from build123d import *

# Parameters (mm, degrees)
F0_R     = 11
F0_R_2   = 10
F0_R_3   = 8.75
F0_R_4   = 7.25
F0_R_5   = 3.5
F0_R_6   = 2.75
F1_DEPTH = 2
F2_DEPTH = 4.25
F3_DEPTH = 12


with BuildPart() as f1:
    # F0 (on Top) → F1 (new body)
    with BuildSketch(Plane.XY):
        Circle(F0_R)
        Circle(F0_R_2, mode=Mode.SUBTRACT)
        Circle(F0_R_2)
        Circle(F0_R_3, mode=Mode.SUBTRACT)
        Circle(F0_R_3)
        Circle(F0_R_4, mode=Mode.SUBTRACT)
        Circle(F0_R_4)
        Circle(F0_R_5, mode=Mode.SUBTRACT)
        Circle(F0_R_5)
        Circle(F0_R_6, mode=Mode.SUBTRACT)
    extrude(amount=F1_DEPTH)

    # F0 (on Top) → F2 (join)
    with BuildSketch(Plane.XY):
        Circle(F0_R_5)
        Circle(F0_R_6, mode=Mode.SUBTRACT)
    extrude(amount=-F2_DEPTH)

    # F0 (on Top) → F3 (join)
    with BuildSketch(Plane.XY):
        Circle(F0_R_2)
        Circle(F0_R_3, mode=Mode.SUBTRACT)
    extrude(amount=F3_DEPTH)


solid = f1.part
Part model, mm, in its own coordinate system. A direction names the side the tool comes from. Coordinates: 2 decimals unless noted, no trailing zeros. Order: outer loops, then holes, each group sorted by start corner. A loop starts at its lowest first (then second) coordinate and runs counter-clockwise, first axis right, second up. Notation, with made-up numbers: M 17.5,-37 L 43.5,-37 A25 ccw 43.5,-9 Z; hole C 0.5,57 d5. An arc over 180 degrees is marked long. Use a Markdown table: item, result.
(1) Cut at D-D on x = 6. Write the cut outline in (y, z).
A:
| item | result |
|---|---|
| outline | M -9.22,0 L 9.22,0 L 9.22,2 L 8,2 L 8,12 L 6.37,12 L 6.37,2 L -6.37,2 L -6.37,12 L -8,12 L -8,2 L -9.22,2 Z |
(2) Cut at A-A on y = 0. Write the cut outline in (x, z).
A:
| item | result |
|---|---|
| outline | M -11,0 L -3.5,0 L -3.5,-4.25 L -2.75,-4.25 L -2.75,2 L -8.75,2 L -8.75,12 L -10,12 L -10,2 L -11,2 Z; M 2.75,-4.25 L 3.5,-4.25 L 3.5,0 L 11,0 L 11,2 L 10,2 L 10,12 L 8.75,12 L 8.75,2 L 2.75,2 Z |
(3) Probe L1, parallel to Y at x = 0, z = 0.5; L2, parallel to X at y = 0, z = 5. List the from-to ranges inside material, lowest first.
A:
| item | result |
|---|---|
| L1 | y = -11 to -2.75, 2.75 to 11 |
| L2 | x = -10 to -8.75, 8.75 to 10 |
(4) Cut at C-C on z = 11. Write the cut outline in (x, y).
A:
| item | result |
|---|---|
| outline | C 0,0 d20; hole C 0,0 d17.5 |
(5) Flat gauge pins, fed straight in: pin 1 (4 mm diameter, centred on x = 0, y = 5, fed in from +Z); pin 2 (4 mm diameter, centred on y = 6.5, z = 7, fed in from +X); pin 3 (6 mm diameter, centred on y = -1.5, z = 8.5, fed in from +X). Where does each tip first touch, or does it go through?
A:
| item | result |
|---|---|
| pin 1 | stops at z = 2 |
| pin 2 | stops at x = 8.93 |
| pin 3 | stops at x = 10 |
(6) Pull direction X, two halves, no side cores. Call faces 1 (the cylindrical face through (3.233, -1.341, -2.095)), 2 (the cylindrical face through (-6.944, -5.324, 6.93)), 3 (the flat face through (-3, -1, -4.25)): released by +X, released by -X, zero draft, split by the parting line, or undercut.
A:
| item | result |
|---|---|
| face 1 | split by the parting line |
| face 2 | undercut |
| face 3 | zero draft |
(7) Tool access for faces 4 (the flat face through (-3, 3, 0)), 5 (the cylindrical face through (-2.17, -9.76, 6.93)), 6 (the flat face through (0, -9, 12)): list every direction of +Z, -Z, +X, -X, +Y, -Y with a clear straight run to the whole face (end or side of a thin tool).
A:
| item | result |
|---|---|
| face 4 | -Z |
| face 5 | +Z |
| face 6 | +Z, +X, -X, +Y, -Y |
